from build123d import *

# Parameters (mm, degrees)
ESQUISSE1_W             = 5
ESQUISSE1_H             = 5
BOSS_EXTRU_1_DEPTH      = 2
ENL_V_MAT_EXTRU_1_DEPTH = 6
ESQUISSE3_R             = 1
BOSS_EXTRU_2_DEPTH      = 20
ESQUISSE4_W             = 1
ESQUISSE4_H             = 0.2
CONG_3_R                = 0.3


with BuildPart() as part:
    # Esquisse1 → Boss.-Extru.1 (new body, symmetric)
    with BuildSketch(Plane(origin=(0, 0, 0), x_dir=(1, 0, 0), z_dir=(0, 1, 0))):
        Rectangle(ESQUISSE1_W, ESQUISSE1_H)
    extrude(amount=BOSS_EXTRU_1_DEPTH, both=True)

    # Esquisse2 → Enlèv. mat.-Extru.1 (cut, through all)
    with BuildSketch(Plane.ZY.offset(2.5)):
        Polygon((2.5, 2), (1.345299462, 0), (2.5, -2), align=None)
    extrude(amount=-ENL_V_MAT_EXTRU_1_DEPTH, mode=Mode.SUBTRACT)

    # Esquisse3 → Boss.-Extru.2 (add)
    with BuildSketch(Plane(origin=(0, 0, -2.5), x_dir=(-1, 0, 0), z_dir=(0, 0, -1))):
        Circle(ESQUISSE3_R)
    extrude(amount=BOSS_EXTRU_2_DEPTH)

    # Esquisse4 → Enlèvement de matière-Révolution1 (revolve, cut)
    with BuildSketch(Plane(origin=(0, 0, 0), x_dir=(0, 0, -1), z_dir=(1, 0, 0))):
        with Locations((21.5, 0.9)):
            Rectangle(ESQUISSE4_W, ESQUISSE4_H)
    revolve(axis=Axis((0, 0, -23.5), (0, 0, -1)), mode=Mode.SUBTRACT)

    # Congé3
    cong_3_edges = [part.edges().sort_by_distance(p)[0] for p in [
        (-2.5, 2, 0),
        (0, 2, 2.5),
        (2.5, -1, 1.922649731),
        (2.5, 1, 1.922649731),
        (0, 0, 1.345299462),
        (-2.5, 1, 1.922649731),
        (-2.5, -1, 1.922649731),
        (1, 0, -2.5),
        (2.5, 2, 0),
        (0, -2, 2.5),
        (-2.5, -2, 0),
        (0, -2, -2.5),
        (2.5, -2, 0),
        (-2.5, 0, -2.5),
        (2.5, 0, -2.5),
        (0, 2, -2.5),
    ]]
    fillet(cong_3_edges, radius=CONG_3_R)


solid = part.part
Geometry check sheet. Reference: the model listing, model coordinates, mm. A direction names the side the tool comes from. Round coordinates to 2 decimals unless told otherwise and drop trailing zeros. Loops run counter-clockwise (first coordinate to the right, second up) from the corner with the lowest first, then second, coordinate; pieces in that order, holes last.
Item 1: Gauge pin test, flat ends, axial feed: pin 1 (1 mm diameter, centred on x = 0.5, y = 0, fed in from +Z); pin 2 (2 mm diameter, centred on x = 0, z = -13, fed in from +Y); pin 3 (2 mm diameter, centred on x = 0.5, y = 0.5, fed in from +Z). Record the tip position at first contact, or that the pin passes through.
Item 2: Thickness scan on line 1 (X direction, y = -0.1, z = -16.75); line 2 (Z direction, x = 1.35, y = 1.1); line 3 (Y direction, x = -0.2, z = -7). Record the ranges inside material, lowest first.
Item 3: Cross-section at C-C on x = 1.9. Record the boundary of the cut face in (y, z), then the cut area to 3 significant figures.
Item 4: Cross-section at B-B on z = -18.5. Record the boundary of the cut face in (x, y).
Item 5: Cross-section at A-A on x = 0. Record the boundary of the cut face in (y, z).
Item 6: Mould release check, pull along Z, two halves, no side actions. Record for faces 1 (the flat face through (0, 2, 0)), 2 (the flat face through (0, 0, -22.5)), 3 (the cylindrical face through (-0.49, -0.63, -21.51)), 4 (the cylindrical face through (-2.414, 0.885, 1.752)): pulls with the +Z half, pulls with the -Z half, needs draft (parallel to the pull), parting line crosses it, or undercut.
Item 7: Access from +Z, -Z, +X, -X, +Y, -Y to the whole of each face (thin tool, end or side, straight path). Record for faces 5 (the flat face through (-0.03, 0.86, 1.84)), 6 (the cylindrical face through (2.414, -0.885, 1.752)), 7 (the cylindrical face through (-2.414, -0.905, 1.764)), 8 (the cylindrical face through (-1, 0, -12)).
Answer sheet:
1. pin 1: stops at z = 1.63
1. pin 2: stops at y = 1
1. pin 3: stops at z = 2.21
2. line 1: x = -0.99 to 0.99
2. line 2: z = -2.5 to 1.98
2. line 3: y = -0.98 to 0.98
3. outline: (-2, -2.2) arc R0.3 ccw to (-1.7, -2.5) - (1.7, -2.5) arc R0.3 ccw to (2, -2.2) - (2, 1.98) arc R0.3 ccw to (1.55, 2.24) - (0.15, 1.43) arc R0.3 cw to (-0.15, 1.43) - (-1.55, 2.24) arc R0.3 ccw to (-2, 1.98) - close
3. area: 17.5 mm2
4. outline: circle Ø2 at (0, 0)
5. outline: (-2, -2.2) arc R0.3 ccw to (-1.7, -2.5) - (-1.3, -2.5) arc R0.3 cw to (-1, -2.8) - (-1, -21) - (-0.8, -21) - (-0.8, -22) - (-1, -22) - (-1, -22.5) - (1, -22.5) - (1, -22) - (0.8, -22) - (0.8, -21) - (1, -21) - (1, -2.8) arc R0.3 cw to (1.3, -2.5) - (1.7, -2.5) arc R0.3 ccw to (2, -2.2) - (2, 1.98) arc R0.3 ccw to (1.55, 2.24) - (0.15, 1.43) arc R0.3 cw to (-0.15, 1.43) - (-1.55, 2.24) arc R0.3 ccw to (-2, 1.98) - close
6. face 1: needs draft
6. face 2: pulls with the -Z half
6. face 3: undercut
6. face 4: pulls with the +Z half
7. face 5: +Z, +X, -X
7. face 6: +Z, +X
7. face 7: +Z, -X
7. face 8: -Z
